Autodesk Inventor part; units mm, degrees
ref_plane "YZ Plane" through (0, 0, 0) normal (1, 0, 0) x (0, 1, 0)
ref_plane "XZ Plane" through (0, 0, 0) normal (0, 1, 0) x (-1, 0, 0)
ref_plane "XY Plane" through (0, 0, 0) normal (0, 0, 1) x (1, 0, 0)
sketch "Sketch1" plane through (0, 0, 0) normal (0, 0, 1) x (1, 0, 0)
  line L0 (-40.64, 12.7) -> (40.64, 12.7)
  line L1 (40.64, 12.7) -> (40.64, -12.7)
  line L2 (40.64, -12.7) -> (-40.64, -12.7)
  line L3 (-40.64, -12.7) -> (-40.64, 12.7)
  point P0 (0, 0)
  dimension "d0" = 81.28
  dimension "d1" = 40.64
  dimension "d2" = 12.7
  dimension "d3" = 25.4
extrude "Extrusion1" add sketch "Sketch1" along normal mid plane 6.35
sketch "Sketch2" plane through (0, 0, 3.175) normal (0, 0, 1) x (1, 0, 0)
  circle A0 centre (-23.7067, 0) radius 11.303
  circle A1 centre (0, 0) radius 11.303
  line L0 (40.64, -12.7) -> (40.64, 12.7)
  circle A2 centre (23.7067, 0) radius 11.303
  line L1 (-40.64, 12.7) -> (-40.64, -12.7)
  line L2 (-40.64, 0) -> (40.64, 0) construction
  line L3 (40.64, 12.7) -> (-40.64, 12.7)
  point P0 (0, 0)
  dimension "d6" = 22.606
  dimension "d9" = 22.606
  dimension "d11" = 22.606
  dimension "d14" = 23.7067
  dimension "d21" = 81.28
  dimension "d22" = 23.7067
  dimension "d45" = 0
sketch "Sketch4" plane through (-40.64, -12.7, -3.175) normal (-1, 0, 0) x (0, 0, 1)
  line L0 (0, 0) -> (0, 25.4)
  line L1 (6.35, 25.4) -> (6.35, 0)
  line L2 (0, 16.51) -> (6.35, 16.51)
  line L3 (6.35, 16.51) -> (6.35, 8.89)
  line L4 (6.35, 8.89) -> (0, 8.89)
  line L5 (0, 8.89) -> (0, 16.51)
  point P0 (3.175, 12.7)
  point P1 (0, 25.4)
  dimension "d30" = 3.81
  dimension "d31" = 7.62
extrude "Extrusion3" cut sketch "Sketch4" against normal blind 0.635
mirror "Mirror1" about plane through (0, 0, 0) normal (1, 0, 0) of "Extrusion3"
sketch "Sketch5" plane through (0, 0, 3.175) normal (0, 0, 1) x (1, 0, 0)
  circle A0 centre (0, 8.128) radius 3.175 construction
  line L0 (40.64, 12.7) -> (-40.64, 12.7)
  line L1 (-22.0846, 0) -> (40.005, 0) construction
  line L2 (40.005, 3.81) -> (40.005, -3.81)
  circle A1 centre (0, -8.128) radius 3.175 construction
  circle A2 centre (-36.068, 8.128) radius 3.175
  circle A3 centre (36.068, -8.128) radius 3.175
  line L3 (-40.64, 12.7) -> (-40.64, 3.81)
  line L4 (40.64, -3.81) -> (40.64, -12.7)
  line L5 (40.64, -12.7) -> (-40.64, -12.7)
  point P0 (0, 0)
  dimension "d34" = 6.35
  dimension "d35" = 4.572
  dimension "d48" = 6.35
  dimension "d49" = 6.35
  dimension "d50" = 4.572
  dimension "d51" = 4.572
  dimension "d52" = 4.572
  dimension "d53" = 4.572
extrude "Extrusion4" cut sketch "Sketch5" against normal blind 1.27
sketch "Sketch7" plane through (-40.64, -12.7, 3.175) normal (0, -1, 0) x (1, 0, 0)
  line L0 (26.67, -14.605) -> (54.61, -14.605)
  line L1 (54.61, -14.605) -> (54.61, 8.255)
  line L2 (54.61, 8.255) -> (26.67, 8.255)
  line L3 (26.67, 8.255) -> (26.67, -14.605)
  point P0 (40.64, -3.175)
  dimension "d39" = 27.94
  dimension "d40" = 22.86
  dimension "d41" = 11.43
  dimension "d42" = 13.97
extrude "Extrusion5" [suppressed]
extrude "Extrusion6" cut sketch "Sketch2" against normal blind 25.4
sketch "Sketch8" plane through (0, 0, -3.175) normal (0, 0, -1) x (-1, 0, 0)
  line L0 (40.005, 3.81) -> (40.005, -3.81) construction
  line L1 (40.005, 0) -> (-40.005, 0)
  line L2 (-40.005, 3.81) -> (-40.005, -3.81) construction
  line L3 (40.64, 12.7) -> (-40.64, 12.7)
  line L4 (40.64, 3.81) -> (40.64, 12.7)
  line L5 (-40.64, 12.7) -> (-40.64, 3.81)
  line L6 (-40.005, 3.81) -> (-40.005, 0)
  line L7 (-40.64, 3.81) -> (-40.005, 3.81)
  line L8 (40.005, 3.81) -> (40.005, 0)
  line L9 (40.005, 3.81) -> (40.64, 3.81)
  point P0 (0, 0)
extrude "Extrusion7" [suppressed]
sketch "Sketch9" plane through (0, 0, -3.175) normal (0, 0, -1) x (-1, 0, 0)
  line L0 (-40.64, -12.7) -> (40.64, -12.7)
  line L1 (40.64, -12.7) -> (40.64, -3.81)
  line L2 (40.64, -3.81) -> (40.005, -3.81)
  line L3 (-40.005, -3.81) -> (-40.64, -3.81)
  line L4 (-40.64, -3.81) -> (-40.64, -12.7)
  line L5 (-40.005, 3.81) -> (-40.005, -3.81)
  line L6 (-40.005, 0) -> (-40.005, -3.81)
  line L7 (-40.005, 0) -> (40.005, 0)
  line L8 (40.005, -3.81) -> (40.005, 3.81)
  line L9 (40.005, -3.81) -> (40.005, 0)
  point P0 (0, 0)
extrude "Extrusion8" [suppressed]
equation "\"d9\" = d7"
equation "\"d11\" = d9"
equation "\"d22\" = d14"
equation "\"d7\" = d6"
properties part number "Tube Holder" material "Aluminum 6061-AHC"
Check sheet for the modelled part. Datum: model origin and axes. Units: mm. A direction names the side the tool comes from. Give positions to 0.01 mm unless a question says otherwise; leave off trailing zeros. Write each loop counter-clockwise with the first axis right and the second up, starting at its lowest first coordinate (ties: lowest second). Pieces come first, ordered by that corner, then holes. Notation, with made-up numbers: (44, 85.25) - (75, 85.25) arc R17 ccw to (75, 99.25) - close; hole circle Ø7 at (10, 86.25). An arc over 180 degrees is marked (long way). Answer as a JSON object with one key per item and string values. Group by question number.
1) Thickness scan on probe 1 along X at (y, z) = (5.25, -2); probe 2 along X at (y, z) = (7.25, 0.25); probe 3 along Y at (x, z) = (-16, -2.5). Record the ranges inside material, lowest first. Write a range as from..to.
2) Sectioned sample at B-B (y = 0). Record the cut outline in (x, z) (3 decimals), then the cut area to 3 significant figures.
3) Sectioned sample at A-A (x = 0). Record the cut outline in (y, z) (3 decimals), then the cut area to 3 significant figures.
4) Sectioned sample at C-C (z = -1.75). Record the cut outline in (x, y) (3 decimals).
5) Release check for a two-part mould opening along X. For faces 3 (the face through (-40.005, 0, 0)), 4 (the face through (36, -8, 1.905)), 5 (the face through (40.005, 0, 0)), 6 (the face through (39.001, -9.344, 2.549)) record: pulls with the +X half, pulls with the -X half, needs draft (parallel to the pull), parting line crosses it, or undercut.
6) Access from +Z, -Z, +X, -X, +Y, -Y to the whole of each face (thin tool, end or side, straight path). Record for faces 1 (the face through (-0.6, 11.5, -3.175)), 2 (the face through (-33.04, 9.08, 2.55)).
7) Sectioned sample at D-D (x = -21). Record the cut outline in (y, z) (3 decimals).
8) Depth check by flat-ended pin: P1, Ø3, axis at x = -37, y = 8.5, coming from the +Z side (3 decimals); P2, Ø3, axis at y = 1, z = -1.5, coming from the -X side (3 decimals); P3, Ø3, axis at y = 2, z = 1.5, coming from the +X side (3 decimals). Enter the tip coordinate at first touch or a pass-through.
Geometry results:
{
 "1": {"probe 1": "x = -40.64..-33.72, -13.7..-10.01, 10.01..13.7, 33.72..40.64", "probe 2": "x = -40.64..-32.38, -15.04..-8.67, 8.67..15.04, 32.38..40.64", "probe 3": "y = -12.7..-8.27, 8.27..12.7"},
 "2": {"outline": "(-40.005, -3.175) - (-35.01, -3.175) - (-35.01, 3.175) - (-40.005, 3.175) - close; (-12.404, -3.175) - (-11.303, -3.175) - (-11.303, 3.175) - (-12.404, 3.175) - close; (11.303, -3.175) - (12.404, -3.175) - (12.404, 3.175) - (11.303, 3.175) - close; (35.01, -3.175) - (40.005, -3.175) - (40.005, 3.175) - (35.01, 3.175) - close", "area": "77.4 mm^2"},
 "3": {"outline": "(-12.7, -3.175) - (-11.303, -3.175) - (-11.303, 3.175) - (-12.7, 3.175) - close; (11.303, -3.175) - (12.7, -3.175) - (12.7, 3.175) - (11.303, 3.175) - close", "area": "17.7 mm^2"},
 "4": {"outline": "(-40.64, -12.7) - (40.64, -12.7) - (40.64, -3.81) - (40.005, -3.81) - (40.005, 3.81) - (40.64, 3.81) - (40.64, 12.7) - (-40.64, 12.7) - (-40.64, 3.81) - (-40.005, 3.81) - (-40.005, -3.81) - (-40.64, -3.81) - close; hole circle Ø22.606 at (-23.707, 0); hole circle Ø22.606 at (0, 0); hole circle Ø22.606 at (23.707, 0)"},
 "5": {"face 3": "pulls with the -X half", "face 4": "undercut", "face 5": "pulls with the +X half", "face 6": "undercut"},
 "6": {"face 1": "-Z, +X, -X, +Y, -Y", "face 2": "+Z"},
 "7": {"outline": "(-12.7, -3.175) - (-10.974, -3.175) - (-10.974, 3.175) - (-12.7, 3.175) - close; (10.974, -3.175) - (12.7, -3.175) - (12.7, 3.175) - (10.974, 3.175) - close"},
 "8": {"P1": "stops at z = 1.905", "P2": "stops at x = -40.005", "P3": "stops at x = 40.005"}
}
